from build123d import *

# Parameters (mm, degrees)
F0_R     = 1.182239
F0_R_2   = 0.817997
F1_DEPTH = 5.842
F2_DEPTH = 3.81
F3_DEPTH = 5.08
F4_DEPTH = 4.318
F5_R     = 1.905
F6_DEPTH = 25.4
F7_DEPTH = 6.35


with BuildPart() as f1:
    # F0 (on Front) → F1 (new body)
    with BuildSketch(Plane.XZ):
        Polygon((-4.180855, -20.625193), (-4.353608, -20.920252), (-3.424949, -21.167446), (-3.28061, -20.625193), align=None)
        Polygon((3.424949, -21.167446), (4.353608, -20.920252), (4.180855, -20.625193), (3.28061, -20.625193), align=None)
        Polygon((22.26289, -6.835999), (22.26289, 1.657223), (4.394875, -5.754956), (2.197438, -5.957079), (0, -6.159202), (-2.197438, -5.957079), (-4.394875, -5.754956), (-22.26289, 1.657223), (-22.26289, -6.835999), (-22.832444, -9.118818), (-15.86828, -11.246894), (-14.217053, -15.145346), (-4.353608, -20.920252), (-4.180855, -20.625193), (-4.180855, -11.195441), (-3.601368, -9.465247), (0, -9.465247), (3.601368, -9.465247), (4.180855, -11.195441), (4.180855, -20.625193), (4.353608, -20.920252), (14.217053, -15.145346), (15.86828, -11.246894), (22.832444, -9.118818), align=None)
        Polygon((-15.86828, -11.246894), (-22.832444, -9.118818), (-22.26289, -10.434624), (-14.217053, -15.145346), align=None)
        Polygon((22.26289, -10.434624), (22.832444, -9.118818), (15.86828, -11.246894), (14.217053, -15.145346), align=None)
        Polygon((24.816887, 1.657223), (22.26289, 1.657223), (22.26289, -6.835999), (22.832444, -9.118818), (25.498668, -5.754956), align=None)
        with Locations((23.784082, -3.675047)):
            Circle(F0_R, mode=Mode.SUBTRACT)
        with Locations((23.597831, -0.42893)):
            Circle(F0_R_2, mode=Mode.SUBTRACT)
        Polygon((-22.26289, -6.835999), (-22.26289, 1.657223), (-24.816887, 1.657223), (-25.498668, -5.754956), (-22.832444, -9.118818), align=None)
        with Locations((-23.784082, -3.675047)):
            Circle(F0_R, mode=Mode.SUBTRACT)
        with Locations((-23.597831, -0.42893)):
            Circle(F0_R_2, mode=Mode.SUBTRACT)
        Polygon((-19.404403, 16.750786), (-22.26289, 15.816627), (-23.496922, 2.400486), (-22.26289, 1.657223), align=None)
        Polygon((23.496922, 2.400486), (22.26289, 15.816627), (19.404403, 16.750786), (22.26289, 1.657223), align=None)
        Polygon((24.816887, 1.657223), (23.496922, 2.400486), (22.26289, 1.657223), align=None)
        Polygon((-22.26289, 1.657223), (-23.496922, 2.400486), (-24.816887, 1.657223), align=None)
        Polygon((-19.404403, 16.750786), (-22.832444, 16.386179), (-22.26289, 15.816627), align=None)
        Polygon((22.26289, 15.816627), (22.832444, 16.386179), (19.404403, 16.750786), align=None)
        Polygon((22.832444, 16.386179), (22.136323, 20.879321), (5.009265, 22.700958), (2.695112, 21.684956), (0, 21.684956), (-2.695112, 21.684956), (-5.009265, 22.700958), (-22.136323, 20.879321), (-22.832444, 16.386179), (-19.404403, 16.750786), (-5.009265, 18.281856), (-2.695112, 17.265854), (0, 17.265854), (2.695112, 17.265854), (5.009265, 18.281856), (19.404403, 16.750786), align=None)
        Polygon((3.467637, 26.608711), (0, 26.608711), (-3.467637, 26.608711), (-4.353608, 27.524108), (-12.96019, 26.608711), (-16.187659, 24.61306), (-16.630644, 23.537237), (-22.136323, 20.879321), (-5.009265, 22.700958), (-2.695112, 21.684956), (0, 21.684956), (2.695112, 21.684956), (5.009265, 22.700958), (22.136323, 20.879321), (16.630644, 23.537237), (16.187659, 24.61306), (12.96019, 26.608711), (4.353608, 27.524108), align=None)
    extrude(amount=F1_DEPTH)

    # F0 (on Front) → F2 (join)
    with BuildSketch(Plane.XZ):
        with Locations((23.784082, -3.675047)):
            Circle(F0_R)
        with Locations((23.597831, -0.42893)):
            Circle(F0_R_2)
        with Locations((-23.784082, -3.675047)):
            Circle(F0_R)
        with Locations((-23.597831, -0.42893)):
            Circle(F0_R_2)
        Polygon((22.26289, 1.657223), (19.404403, 16.750786), (18.012892, 15.012917), (13.572707, 15.012917), (11.013955, 13.131482), (5.896451, 13.131482), (4.394875, 15.088174), (0, 15.088174), (-4.394875, 15.088174), (-5.896451, 13.131482), (-11.013955, 13.131482), (-13.572707, 15.012917), (-18.012892, 15.012917), (-19.404403, 16.750786), (-22.26289, 1.657223), (-4.394875, -5.754956), (-2.197438, -5.957079), (-1.331172, -3.868833), (0, -3.868833), (1.331172, -3.868833), (2.197438, -5.957079), (4.394875, -5.754956), align=None)
        Polygon((-2.750259, 0), (-4.015016, -3.048861), (-11.364689, 0), (-11.364689, 3.272761), (-7.025312, 8.089235), (-4.015016, 8.089235), (-1.832551, 11.701591), (0, 11.701591), (1.832551, 11.701591), (4.015016, 8.089235), (7.025312, 8.089235), (11.364689, 3.272761), (11.364689, 0), (4.015016, -3.048861), (2.750259, 0), (0, 0), align=None, mode=Mode.SUBTRACT)
    extrude(amount=F2_DEPTH)

    # F0 (on Front) → F3 (join)
    with BuildSketch(Plane.XZ):
        Polygon((0, -6.159202), (2.197438, -5.957079), (1.331172, -3.868833), (0, -3.868833), (-1.331172, -3.868833), (-2.197438, -5.957079), align=None)
    extrude(amount=F3_DEPTH)

    # F0 (on Front) → F4 (join)
    with BuildSketch(Plane.XZ):
        Polygon((-11.364689, 0), (-4.015016, -3.048861), (-2.750259, 0), (0, 0), (2.750259, 0), (4.015016, -3.048861), (11.364689, 0), (11.364689, 3.272761), (7.025312, 8.089235), (4.015016, 8.089235), (1.832551, 11.701591), (0, 11.701591), (-1.832551, 11.701591), (-4.015016, 8.089235), (-7.025312, 8.089235), (-11.364689, 3.272761), align=None)
        Polygon((18.012892, 15.012917), (19.404403, 16.750786), (5.009265, 18.281856), (2.695112, 17.265854), (0, 17.265854), (-2.695112, 17.265854), (-5.009265, 18.281856), (-19.404403, 16.750786), (-18.012892, 15.012917), (-13.572707, 15.012917), (-11.013955, 13.131482), (-5.896451, 13.131482), (-4.394875, 15.088174), (0, 15.088174), (4.394875, 15.088174), (5.896451, 13.131482), (11.013955, 13.131482), (13.572707, 15.012917), align=None)
    extrude(amount=F4_DEPTH)

    # F5 (on face) → F6 (cut)
    with BuildSketch(Plane.XZ.offset(5.842)):
        with Locations((0, 24.332419)):
            Circle(F5_R)
    extrude(amount=-F6_DEPTH, mode=Mode.SUBTRACT)

    # F0 (on Front) → F7 (join)
    with BuildSketch(Plane.XZ):
        Polygon((3.28061, -20.625193), (4.180855, -20.625193), (4.180855, -11.195441), (3.601368, -9.465247), (0, -9.465247), (-3.601368, -9.465247), (-4.180855, -11.195441), (-4.180855, -20.625193), (-3.28061, -20.625193), (0, -20.625193), align=None)
    extrude(amount=F7_DEPTH)


solid = f1.part
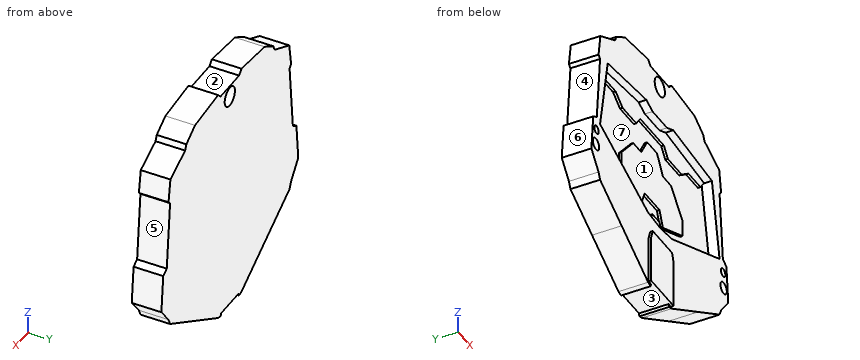
Can you work these out from the model? Positions are in its coordinate system, mm. Face numbers are marked on the shaded views. A direction names the side the tool comes from. Coordinates: 2 decimals unless noted, no trailing zeros. Loops run counter-clockwise (first coordinate to the right, second up) from the corner with the lowest first, then second, coordinate; pieces in that order, holes last. Notation, with made-up numbers: M 16.25,17 L 30.25,17 A25 cw 30.25,40 Z; hole C -23,48 d10. An arc over 180 degrees is marked long. Answer as CSV lines item,"result". Start each with the question number.
1. If I drill on probe 1 along Z at (x, y) = (0, -2.7); probe 2 along Y at (x, z) = (-20, 2.5); probe 3 along Y at (x, z) = (11, -4), over which ranges is the centre line in solid material (lowest first)? Write a range as [from, to].
2. For the marked faces 5, 6 and 7, which set-ups out of +Z, -Z, +X, -X, +Y, -Y let a thin tool reach every point of the face, with its end or its side?
3. For pin 1 Ø1.3 at (x, z) = (23.6, -0.43) entering from -Y; pin 2 Ø3 at (x, y) = (0, -2) entering from -Z; pin 3 Ø3 at (y, z) = (-2, 19) entering from -X, each with a flat end and sliding along its axis, tell me the tip position at first contact or that it passes through.
4. Thinking about a two-plate mould opening in Z: for the marked faces 1, 2, 3 and 4, which applies, +Z half, -Z half, draft (parallel to the pull), parting line (faces both ways), or undercut?
5. Suppose I cut it at B-B, the plane x = 15.5. List the corners of the cut face in (y, z) for me.
6. Suppose I cut it at C-C, the plane x = -10. List the corners of the cut face in (y, z) for me.
7. Suppose I cut it at A-A, the plane z = -13. List the corners of the cut face in (x, y) for me, plus the area to 3 significant figures.
Output:
1,probe 1,"z = [-20.63, 22.43], [26.24, 26.61]"
1,probe 2,"y = [-3.81, 0]"
1,probe 3,"y = [-5.84, 0]"
2,face 5,"+X, +Y, -Y"
2,face 6,"+Z, -X, +Y, -Y"
2,face 7,"-Y"
3,pin 1,"stops at y = -3.81"
3,pin 2,"stops at z = -20.63"
3,pin 3,"stops at x = -22.66"
4,face 1,"undercut"
4,face 2,"+Z half"
4,face 3,"-Z half"
4,face 4,"undercut"
5,outline,"M -5.84,-14.39 L 0,-14.39 L 0,25.04 L -5.84,25.04 L -5.84,17.17 L -4.32,17.17 L -4.32,15.01 L -3.81,15.01 L -3.81,-1.15 L -5.84,-1.15 Z"
6,outline,"M -5.84,-17.61 L 0,-17.61 L 0,26.92 L -5.84,26.92 L -5.84,17.75 L -4.32,17.75 L -4.32,13.13 L -3.81,13.13 L -3.81,4.79 L -4.32,4.79 L -4.32,-0.57 L -3.81,-0.57 L -3.81,-3.43 L -5.84,-3.43 Z"
7,outline,"M -17.88,-5.84 L -4.18,-5.84 L -4.18,-6.35 L 4.18,-6.35 L 4.18,-5.84 L 17.88,-5.84 L 17.88,0 L -17.88,0 Z"
7,area,"213 mm^2"
